Verification items for the finished model (mm, model axes). A direction names the side the tool comes from. Round coordinates to 2 decimals unless told otherwise and drop trailing zeros. Order: outer loops, then holes, each group sorted by start corner. A loop starts at its lowest first (then second) coordinate and runs counter-clockwise, first axis right, second up. Notation, with made-up numbers: (19.5, 50) -> (54.5, 50) arc R10 ccw to (54.5, 61) -> close; hole circle Ø2 at (51.5, 78.25). An arc over 180 degrees is marked (long way). Return JSON: item names as keys, results as strings. Group by question number.
1) Draft check along Z on faces 1 (the flat face through (-7, -30.135, 9)), 2 (the flat face through (-2, -13, -1.27)), 3 (the flat face through (-2, -13, 0)). Enter one of: pulls with the +Z half, pulls with the -Z half, needs draft (parallel to the pull), parting line crosses it, or undercut.
2) Depth check by flat-ended pin: pin 1 (1.7 mm diameter, centred on x = -137.03, y = -3.625, fed in from -Z) (3 decimals); pin 2 (4 mm diameter, centred on x = -105.79, z = 8.25, fed in from +Y); pin 3 (5 mm diameter, centred on x = -33, z = 14, fed in from +Y) (3 decimals); pin 4 (3.5 mm diameter, centred on x = -137.03, y = 6.535, fed in from +Z). Enter the tip coordinate at first touch or a pass-through.
3) Section check B-B on y = 25. Enter the section's corners in (x, z), plus the area to 3 significant figures.
4) Scan lines: L1, parallel to X at y = -29.9, z = 8.25; L2, parallel to Y at x = -96.5, z = 7.5 (3 decimals); L3, parallel to Y at x = 107.08, z = -0.65 (3 decimals). Record each from-to range of solid material in increasing order.
5) Section check A-A on x = -79.5. Enter the section's corners in (y, z) (3 decimals).
6) Tool access check on faces 4 (the flat face through (-143.89, -9.5, -0.4)), 5 (the flat face through (-7.4, -28.865, 8.7)). Record the directions out of +Z, -Z, +X, -X, +Y, -Y that give a thin tool (end or side, any length) a straight path to the whole face; none if there is none.
```python
from build123d import *

# Parameters (mm, degrees)
SKETCH2_W                     = 287.78
SKETCH2_H                     = 60.27
SKETCH2_W_2                   = 233.19
SKETCH2_H_2                   = 28.58
SKETCH2_W_3                   = 18.27
BASE_FLANGE1_DEPTH            = 1.27
EDGE_FLANGE1_STRIP_W          = 6.5532
EDGE_FLANGE1_STRIP_H          = 1.27
EDGE_FLANGE1_STRIP_CUT_DEPTH  = 276.86
EDGE_FLANGE1_RELIEF_W         = 7.1882
EDGE_FLANGE1_RELIEF_H         = 0.635
EDGE_FLANGE1_RELIEF_CUT_DEPTH = 1.27
EDGE_FLANGE1_DEPTH            = 276.86
F_34_0_111_DIAMETER_HOLE1_D   = 2.8194
LPATTERN1_COUNT               = 3
LPATTERN1_PITCH               = 101.6
FILLET1_R                     = 2


# Sheet-metal steps are written as plain solids
with BuildPart() as part:
    # Sketch2 → Base-Flange1 (new body)
    with BuildSketch(Plane.XY):
        Rectangle(SKETCH2_W, SKETCH2_H)
        with Locations((-14.595, 1.875)):
            Rectangle(SKETCH2_W_2, SKETCH2_H_2, mode=Mode.SUBTRACT)
        with Locations((121.295, 1.875)):
            Rectangle(SKETCH2_W_3, SKETCH2_H_2, mode=Mode.SUBTRACT)
    extrude(amount=-BASE_FLANGE1_DEPTH)

    # Edge-Flange1 strip (across the edge) → Edge-Flange1 strip cut (cut)
    with BuildSketch(Plane(origin=(-143.89, -30.135, 0), x_dir=(0, 1, 0), z_dir=(1, 0, 0))):
        with Locations((-1.27, -0.635)):
            Rectangle(EDGE_FLANGE1_STRIP_W, EDGE_FLANGE1_STRIP_H)
    extrude(amount=EDGE_FLANGE1_STRIP_CUT_DEPTH, mode=Mode.SUBTRACT)

    # Edge-Flange1 relief (on the sheet) → Edge-Flange1 relief cut (cut)
    with BuildSketch(Plane(origin=(-143.89, -28.1284, 0), x_dir=(0, 1, 0), z_dir=(0, 0, 1))):
        with Locations((-2.9591, -277.1775)):
            Rectangle(EDGE_FLANGE1_RELIEF_W, EDGE_FLANGE1_RELIEF_H)
    extrude(amount=-EDGE_FLANGE1_RELIEF_CUT_DEPTH, mode=Mode.SUBTRACT)

    # Edge-Flange1 section (across the edge) → Edge-Flange1 (add)
    with BuildSketch(Plane(origin=(-143.89, -30.135, 0), x_dir=(0, 1, 0), z_dir=(1, 0, 0))):
        with BuildLine():
            Line((0, 0.7366), (0, 16.51))
            Line((0, 16.51), (1.27, 16.51))
            Line((1.27, 16.51), (1.27, 0.7366))
            ThreePointArc((1.27, 0.7366), (1.485745145, 0.215745145), (2.0066, 0))
            Line((2.0066, 0), (2.0066, -1.27))
            ThreePointArc((2.0066, -1.27), (0.587719533, -0.682280467), (0, 0.7366))
        make_face()
    extrude(amount=EDGE_FLANGE1_DEPTH)

    # #34 (0.111) Diameter Hole1 (through all)
    with Locations(Plane.XY):
        with Locations((-137.03, 6.535), (-137.03, -3.625), (107.08, 6.535), (107.08, -3.625)):
            Hole(F_34_0_111_DIAMETER_HOLE1_D / 2)

    # Sketch13 → CSK for #4 Flat Head Machine Screw (100)1 (revolve, cut)
    with BuildSketch(Plane(origin=(97.41, -28.865, 8.25), x_dir=(0, 0, 1), z_dir=(1, 0, 0))):
        Polygon((0, 0), (0, 1.27), (1.63195, 1.27), (1.63195, 1.028358553), (2.8575, 0), align=None)
    csk_for_4_flat_head_machine_screw_100 = revolve(axis=Axis((97.41, -22.515, 8.25), (0, -1, 0)), mode=Mode.SUBTRACT)

    # LPattern1: CSK for #4 Flat Head Machine Screw (100)1 ×3
    with Locations(*[(-i * LPATTERN1_PITCH, 0, 0) for i in range(1, LPATTERN1_COUNT)]):
        add(csk_for_4_flat_head_machine_screw_100, mode=Mode.SUBTRACT)

    # Fillet1
    fillet1_edges = [part.edges().sort_by_distance(p)[0] for p in [
        (-143.89, -29.5, 16.51),
        (132.97, -29.5, 16.51),
        (-143.89, 30.135, -0.635),
        (143.89, 30.135, -0.635),
    ]]
    fillet(fillet1_edges, radius=FILLET1_R)


solid = part.part
```
Check result:
{
 "1": {"face 1": "needs draft", "face 2": "pulls with the -Z half", "face 3": "pulls with the +Z half"},
 "2": {"pin 1": "through", "pin 2": "y = -29.58", "pin 3": "y = -28.865", "pin 4": "z = 0"},
 "3": {"outline": "(-143.89, -1.27) -> (143.89, -1.27) -> (143.89, 0) -> (-143.89, 0) -> close", "area": "365 mm^2"},
 "4": {"L1": "-143.89 to -107.42, -104.16 to -5.82, -2.56 to 95.78, 99.04 to 132.97", "L2": "-30.135 to -28.865", "L3": "-29.579 to -5.035, -2.215 to 5.125, 7.945 to 30.135"},
 "5": {"outline": "(-30.135, 0.737) arc R2.007 ccw to (-28.128, -1.27) -> (-12.415, -1.27) -> (-12.415, 0) -> (-28.128, 0) arc R0.737 cw to (-28.865, 0.737) -> (-28.865, 16.51) -> (-30.135, 16.51) -> close; (16.165, -1.27) -> (30.135, -1.27) -> (30.135, 0) -> (16.165, 0) -> close"},
 "6": {"face 4": "+Z, -Z, -X, +Y, -Y", "face 5": "+Z, +X, -X, +Y"}
}
